from build123d import *

# Parameters (mm, degrees)
F0_R     = 150
F0_R_2   = 1.75
F0_W     = 14
F0_H     = 50
F1_DEPTH = 3
F2_R     = 1.75
F3_DEPTH = 3
F4_R     = 1.75
F4_R_2   = 10
F5_DEPTH = 3
F6_R     = 1.75
F7_DEPTH = 25
F9_D     = 3.5


# Not quite as in the source:
# - a feature names something its author has since deleted; it is built from what else it names


with BuildPart() as f1:
    # F0 (on Top) → F1 (new body)
    with BuildSketch(Plane.XY):
        Circle(F0_R)
        with Locations((-138, -19)):
            Circle(F0_R_2, mode=Mode.SUBTRACT)
        with Locations((138, -19)):
            Circle(F0_R_2, mode=Mode.SUBTRACT)
        with Locations((-118, 0)):
            Rectangle(F0_W, F0_H, mode=Mode.SUBTRACT)
        with Locations((-138, 19)):
            Circle(F0_R_2, mode=Mode.SUBTRACT)
        with Locations((118, 0)):
            Rectangle(F0_W, F0_H, mode=Mode.SUBTRACT)
        with Locations((138, 19)):
            Circle(F0_R_2, mode=Mode.SUBTRACT)
    extrude(amount=F1_DEPTH)

    # F2 (on face) → F3 (cut, through all)
    with BuildSketch(Plane.XY.offset(3)):
        with Locations((-123.2603204027, 41.3145666106)):
            Circle(F2_R)
        with Locations((-116.3720186201, 57.9443981958)):
            Circle(F2_R)
        with Locations((-86.089285442, 97.4096244325)):
            Circle(F2_R)
        with Locations((-71.8089253168, 108.3673301546)):
            Circle(F2_R)
        with Locations((-36.8563036221, 124.6660053235)):
            Circle(F2_R)
        with Locations((-19.2829754939, 128.5619183744)):
            Circle(F2_R)
        with Locations((19.2829754939, 128.5619183744)):
            Circle(F2_R)
        with Locations((36.8563036221, 124.6660053235)):
            Circle(F2_R)
        with Locations((71.8089253168, 108.3673301546)):
            Circle(F2_R)
        with Locations((86.089285442, 97.4096244325)):
            Circle(F2_R)
        with Locations((116.3720186201, 57.9443981958)):
            Circle(F2_R)
        with Locations((123.2603204027, 41.3145666106)):
            Circle(F2_R)
        Polygon((-126.5058378572, 57.8123947613), (-130.3326721809, 48.5735994362), (-127.3762576769, 47.3490124526), (-123.5494233532, 56.5878077777), align=None)
        Polygon((-105.810936329, 49.2402858763), (-108.767350833, 50.4648728599), (-112.5941851567, 41.2260775348), (-109.6377706526, 40.0014905512), align=None)
        with Locations((-118.0718042549, 48.9069426563)):
            Circle(F2_R)
        Polygon((-86.6365687608, 104.6935764665), (-78.7030353579, 110.7811907566), (-80.6510719308, 113.3199214455), (-88.5846053337, 107.2323071554), align=None)
        with Locations((-77.7997106273, 101.3905568892)):
            Circle(F2_R)
        Polygon((-67.014815921, 95.548806623), (-68.9628524938, 98.0875373119), (-76.8963858967, 91.9999230218), (-74.9483493239, 89.4611923329), align=None)
        Polygon((80.6510719308, 113.3199214455), (78.7030353579, 110.7811907566), (86.6365687608, 104.6935764665), (88.5846053337, 107.2323071554), align=None)
        with Locations((77.7997106273, 101.3905568892)):
            Circle(F2_R)
        Polygon((67.014815921, 95.548806623), (74.9483493239, 89.4611923329), (76.8963858967, 91.9999230218), (68.9628524938, 98.0875373119), align=None)
        Polygon((123.5494233532, 56.5878077777), (127.3762576769, 47.3490124526), (130.3326721809, 48.5735994362), (126.5058378572, 57.8123947613), align=None)
        with Locations((118.0718042549, 48.9069426563)):
            Circle(F2_R)
        Polygon((105.810936329, 49.2402858763), (109.6377706526, 40.0014905512), (112.5941851567, 41.2260775348), (108.767350833, 50.4648728599), align=None)
        Polygon((-25.2036263018, 136.7873430594), (-34.966586373, 134.62294692), (-34.2739796084, 131.4987996972), (-24.5110195372, 133.6631958366), align=None)
        with Locations((-27.6609826613, 124.7706297099)):
            Circle(F2_R)
        Polygon((-21.0479857142, 118.0424597227), (-30.8109457854, 115.8780635833), (-30.1183390208, 112.7539163605), (-20.3553789496, 114.9183124999), align=None)
        Polygon((34.966586373, 134.62294692), (25.2036263018, 136.7873430594), (24.5110195372, 133.6631958366), (34.2739796084, 131.4987996972), align=None)
        with Locations((27.6609826613, 124.7706297099)):
            Circle(F2_R)
        Polygon((30.1183390208, 112.7539163605), (30.8109457854, 115.8780635833), (21.0479857142, 118.0424597227), (20.3553789496, 114.9183124999), align=None)
    extrude(amount=-F3_DEPTH, mode=Mode.SUBTRACT)

    # F4 (on face) → F5 (cut, through all)
    with BuildSketch(Plane.XY.offset(3)):
        with Locations((-15, 142)):
            Circle(F4_R)
        with Locations((15, 142)):
            Circle(F4_R)
        with Locations((0, 119)):
            Circle(F4_R)
        with Locations((0, 135)):
            Circle(F4_R_2)
    extrude(amount=-F5_DEPTH, mode=Mode.SUBTRACT)

    # F6 (on face) → F7 (cut)
    with BuildSketch(Plane.XY.offset(3)):
        Polygon((-105.9872955413, -67.2096212148), (-113.9208289442, -73.2972355049), (-111.9727923714, -75.8359661938), (-104.0392589685, -69.7483519038), align=None)
        with Locations((-103.1359342379, -79.1389857711)):
            Circle(F6_R)
        Polygon((-92.3510395315, -84.9807360374), (-94.2990761043, -82.4420053484), (-102.2326095072, -88.5296196385), (-100.2845729344, -91.0683503274), align=None)
        Polygon((92.3510395315, -84.9807360374), (100.2845729344, -91.0683503274), (102.2326095072, -88.5296196385), (94.2990761043, -82.4420053484), align=None)
        with Locations((103.1359342379, -79.1389857711)):
            Circle(F6_R)
        Polygon((105.9872955413, -67.2096212148), (104.0392589685, -69.7483519038), (111.9727923714, -75.8359661938), (113.9208289442, -73.2972355049), align=None)
        Polygon((111.9727923714, 75.8359661938), (104.0392589685, 69.7483519038), (105.9872955413, 67.2096212148), (113.9208289442, 73.2972355049), align=None)
        with Locations((103.1359342379, 79.1389857711)):
            Circle(F6_R)
        Polygon((94.2990761043, 82.4420053484), (102.2326095072, 88.5296196385), (100.2845729344, 91.0683503274), (92.3510395315, 84.9807360374), align=None)
        Polygon((-92.3510395315, 84.9807360374), (-100.2845729344, 91.0683503274), (-102.2326095072, 88.5296196385), (-94.2990761043, 82.4420053484), align=None)
        with Locations((-103.1359342379, 79.1389857711)):
            Circle(F6_R)
        Polygon((-111.9727923714, 75.8359661938), (-113.9208289442, 73.2972355049), (-105.9872955413, 67.2096212148), (-104.0392589685, 69.7483519038), align=None)
    extrude(amount=-F7_DEPTH, mode=Mode.SUBTRACT)

    # F9 (through all)
    with Locations(Plane.XY.offset(3)):
        with Locations((-25, -47), (25, -47), (25, -113), (-25, -113)):
            Hole(F9_D / 2)


solid = f1.part
The listing builds one solid part. Answer for the finished solid, in the listing's coordinates (mm). Coordinates: 2 decimals unless noted, no trailing zeros. Put each result on its own line as item: value. Start each with the question number.
1. A cutting plane is placed at A-A on z = 2.2. Count the separate pieces of the cut face and the enclosed holes in it, then the cut area to 3 significant figures.
2. For a pull along Y with two mould halves and no side action, classify faces 1 (the cylindrical face through (5.38, 143.43, 1.52)), 2 (the cylindrical face through (-19.527, 148.724, 1.479)), 3 (the flat face through (-2, 2, 3)) as pulls with the +Y half, pulls with the -Y half, needs draft (parallel to the pull), parting line crosses it, or undercut.
3. Flat-ended cylindrical pins translate along their axes: P1, Ø3, axis at x = -103.14, y = -79.14, coming from the -Z side; P2, Ø1.5, axis at x = 37.5, z = 0.5, coming from the +Y side; P3, Ø0.9, axis at x = 120, z = 1, coming from the +Y side. Find the tip coordinate at first contact, or state that the pin passes through.
4. Consider line 1 (X direction, y = -3, z = 0.5); line 2 (Y direction, x = 0, z = 1.95); line 3 (X direction, y = -20.5, z = 1.65). Determine where each line is inside the solid, lowest interval first. Write a range as from..to.
Resolved:
1. separate pieces: 1
1. enclosed holes: 56
1. area: 68,000 mm2
2. face 1: undercut
2. face 2: parting line crosses it
2. face 3: needs draft
3. P1: passes through
3. P2: stops at y = 145.43
3. P3: stops at y = 90.6
4. line 1: x = -149.97..-125, -111..111, 125..149.97
4. line 2: y = -150..117.25, 120.75..125, 145..150
4. line 3: x = -148.59..-138.9, -137.1..-125, -111..111, 125..137.1, 138.9..148.59
